Can you work these out from the model? Positions are in its coordinate system, mm. A direction names the side the tool comes from. Coordinates: 2 decimals unless noted, no trailing zeros. Order: outer loops, then holes, each group sorted by start corner. A loop starts at its lowest first (then second) coordinate and runs counter-clockwise, first axis right, second up. Notation, with made-up numbers: (37, 53.5) -> (92, 53.5) arc R6 ccw to (92, 63.5) -> close; hole circle Ø11 at (-26.75, 24). An arc over 180 degrees is marked (long way). Use a Markdown table: item, result. Add a question column.
1. We'd pull the mould along Y, two halves only. Please class faces 1 (the flat face through (-29.769, -36.446, 4.93)), 2 (the cylindrical face through (34.178, 15.677, 5.07)), 3 (the cylindrical face through (34.18, -44.47, 5.07)), 4 (the flat face through (-2, 14, 10)): pulls with the +Y half, pulls with the -Y half, needs draft (parallel to the pull), parting line crosses it, or undercut.
2. Suppose I cut it at A-A, the plane x = 6.5. List the corners of the cut face in (y, z) for me.
3. For faces 5 (the cylindrical face through (-37.89, 15.6, 5.07)), 6 (the flat face through (-33.318, -15, 5)), which set-ups out of +Z, -Z, +X, -X, +Y, -Y let a thin tool reach every point of the face, with its end or its side?
4. If I drill on line 1 along Y through (x, z) = (20.5, 5.5); line 2 along X through (y, z) = (-6, 1.5); line 3 along X through (y, z) = (13, 2.25), over which ranges is the centre line in solid material (lowest first)? Write a range as from..to.
5. Suppose I cut it at B-B, the plane y = -30. List the corners of the cut face in (x, z) for me.
6. For pin 1 Ø4 at (x, y) = (-33.32, 11.1) entering from -Z, with a flat end and sliding along its axis, tell me the tip position at first contact or that it passes through.
7. Suppose I cut it at D-D, the plane y = 10. List the corners of the cut face in (x, z) for me (1 decimal), then the cut area to 3 significant figures.
8. Suppose I cut it at C-C, the plane z = 1.25. List the corners of the cut face in (x, y) for me, then the cut area to 3 significant figures.
```python
from build123d import *

# Parameters (mm, degrees)
SKETCH1_W           = 75
SKETCH1_H           = 63
SKETCH1_R           = 2.5
BOSS_EXTRUDE1_DEPTH = 10
FILLET1_R           = 5


with BuildPart() as part:
    # Sketch1 → Boss-Extrude1 (new body)
    with BuildSketch(Plane.XY):
        with Locations((-1.818499155, -14.396959459)):
            Rectangle(SKETCH1_W, SKETCH1_H)
        with Locations((-33.318499155, 11.103040541)):
            Circle(SKETCH1_R, mode=Mode.SUBTRACT)
        with Locations((29.681500845, 11.103040541)):
            Circle(SKETCH1_R, mode=Mode.SUBTRACT)
        with Locations((29.681500845, -39.896959459)):
            Circle(SKETCH1_R, mode=Mode.SUBTRACT)
        with Locations((-33.318499155, -39.896959459)):
            Circle(SKETCH1_R, mode=Mode.SUBTRACT)
        Polygon((-33.318499155, 4.103040541), (-26.318499155, 11.103040541), (22.681500845, 11.103040541), (29.681500845, 4.103040541), (29.681500845, -32.896959459), (22.681500845, -39.896959459), (-26.318499155, -39.896959459), (-33.318499155, -32.896959459), align=None, mode=Mode.SUBTRACT)
    extrude(amount=BOSS_EXTRUDE1_DEPTH)

    # Fillet1
    fillet1_edges = [part.edges().sort_by_distance(p)[0] for p in [
        (-39.318499155, 17.103040541, 5),
        (35.681500845, 17.103040541, 5),
        (35.681500845, -45.896959459, 5),
        (-39.318499155, -45.896959459, 5),
    ]]
    fillet(fillet1_edges, radius=FILLET1_R)


solid = part.part
```
Worked out:
| question | item | result |
|---|---|---|
| 1 | face 1 | undercut |
| 1 | face 2 | pulls with the +Y half |
| 1 | face 3 | pulls with the -Y half |
| 1 | face 4 | needs draft |
| 2 | outline | (-45.9, 0) -> (-39.9, 0) -> (-39.9, 10) -> (-45.9, 10) -> close; (11.1, 0) -> (17.1, 0) -> (17.1, 10) -> (11.1, 10) -> close |
| 3 | face 5 | +Z, -Z, -X, +Y |
| 3 | face 6 | +Z, -Z |
| 4 | line 1 | y = -45.9..-39.9, 11.1..17.1 |
| 4 | line 2 | x = -39.32..-33.32, 29.68..35.68 |
| 4 | line 3 | x = -39.24..-34.95, -31.69..28.05, 31.31..35.6 |
| 5 | outline | (-39.32, 0) -> (-33.32, 0) -> (-33.32, 10) -> (-39.32, 10) -> close; (29.68, 0) -> (35.68, 0) -> (35.68, 10) -> (29.68, 10) -> close |
| 6 | pin 1 | passes through |
| 7 | outline | (-39.3, 0) -> (-35.6, 0) -> (-35.6, 10) -> (-39.3, 10) -> close; (-31.1, 0) -> (-27.4, 0) -> (-27.4, 10) -> (-31.1, 10) -> close; (23.8, 0) -> (27.4, 0) -> (27.4, 10) -> (23.8, 10) -> close; (31.9, 0) -> (35.7, 0) -> (35.7, 10) -> (31.9, 10) -> close |
| 7 | area | 148 mm² |
| 8 | outline | (-39.32, -40.9) arc R5 ccw to (-34.32, -45.9) -> (30.68, -45.9) arc R5 ccw to (35.68, -40.9) -> (35.68, 12.1) arc R5 ccw to (30.68, 17.1) -> (-34.32, 17.1) arc R5 ccw to (-39.32, 12.1) -> close; hole circle Ø5 at (-33.32, -39.9); hole circle Ø5 at (-33.32, 11.1); hole (-33.32, -32.9) -> (-26.32, -39.9) -> (22.68, -39.9) -> (29.68, -32.9) -> (29.68, 4.1) -> (22.68, 11.1) -> (-26.32, 11.1) -> (-33.32, 4.1) -> close; hole circle Ø5 at (29.68, -39.9); hole circle Ø5 at (29.68, 11.1) |
| 8 | area | 1,510 mm² |
